```python
from build123d import *

# Parameters (mm, degrees)
SKETCH1_R           = 2.6375
BOSS_EXTRUDE1_DEPTH = 4


with BuildPart() as part:
    # Sketch1 → Boss-Extrude1 (new body)
    with BuildSketch(Plane.XY.offset(4)):
        with BuildLine():
            Line((17.952113198, 57.448352953), (10.955070442, 79.331722279))
            ThreePointArc((10.955070442, 79.331722279), (10.929647665, 81.056262686), (11.867204342, 82.503906776))
            ThreePointArc((11.867204342, 82.503906776), (9.81999759, 91.182758949), (4.022786968, 84.407371171))
            Line((4.022786968, 84.407371171), (3.500292698, 83.52050233))
            Line((3.500292698, 83.52050233), (14.672653681, 49.728262883))
            Line((14.672653681, 49.728262883), (15.200071751, 48.596801815))
            ThreePointArc((15.200071751, 48.596801815), (23.810416572, 47.35893823), (20.452073098, 55.383392934))
            ThreePointArc((20.452073098, 55.383392934), (18.899078146, 56.049025475), (17.952113198, 57.448352953))
        make_face()
        with Locations((19.856196321, 50.419026825)):
            Circle(SKETCH1_R, mode=Mode.SUBTRACT)
        with Locations((8.640951758, 86.323762043)):
            Circle(SKETCH1_R, mode=Mode.SUBTRACT)
    extrude(amount=-BOSS_EXTRUDE1_DEPTH)


solid = part.part
```
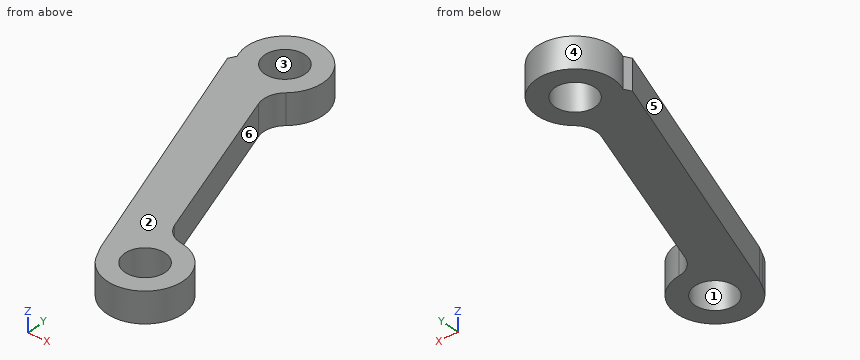
Verification items for the finished model (mm, model axes). Face numbers are marked on the shaded views. A direction names the side the tool comes from. Give positions to 0.01 mm unless a question says otherwise; leave off trailing zeros. Order: outer loops, then holes, each group sorted by start corner. A loop starts at its lowest first (then second) coordinate and runs counter-clockwise, first axis right, second up. Notation, with made-up numbers: M 14,17.5 L 35,17.5 A8 cw 35,26.5 Z; hole C -32.5,4.25 d4. An arc over 180 degrees is marked long. Return JSON: item names as keys, results as strings. Group by question number.
1) Section check C-C on z = 3. Record the cut outline in (x, y) (1 decimal).
2) Go/stop test with flat-tipped pins: pin 1 Ø1.5 at (y, z) = (55.5, 3) entering from -X; pin 2 Ø1.5 at (y, z) = (70.5, 2) entering from -X; pin 3 Ø1.5 at (y, z) = (64, 2) entering from +X. Record where each tip stops, or that it passes through.
3) Mould release check, pull along X, two halves, no side actions. Record for the marked faces 1, 2, 3 and 4: pulls with the +X half, pulls with the -X half, needs draft (parallel to the pull), parting line crosses it, or undercut.
4) Section check D-D on y = 58.5. Record the cut outline in (x, z).
5) Section check A-A on x = 13. Record the cut outline in (y, z), and give its area (3 significant figures).
6) Section check B-B on y = 85.5. Record the cut outline in (x, z).
7) Access from +Z, -Z, +X, -X, +Y, -Y to the whole of each face (thin tool, end or side, straight path). Record for the marked faces 5 and 6.
8) Scan lines: line 1 (X direction, y = 86.5, z = 2.4); line 2 (X direction, y = 85, z = 2); line 3 (Y direction, x = 18.75, z = 3.7). Record each from-to range of solid material in increasing order.
Answer block:
{
 "1": {"outline": "M 3.5,83.5 L 14.7,49.7 L 15.2,48.6 A5 ccw long 20.5,55.4 A3 cw 18,57.4 L 11,79.3 A3 cw 11.9,82.5 A5 ccw long 4,84.4 Z; hole C 8.6,86.3 d5.3; hole C 19.9,50.4 d5.3"},
 "2": {"pin 1": "stops at x = 12.52", "pin 2": "stops at x = 7.56", "pin 3": "stops at x = 16.1"},
 "3": {"face 1": "undercut", "face 2": "needs draft", "face 3": "undercut", "face 4": "parting line crosses it"},
 "4": {"outline": "M 11.77,0 L 17.62,0 L 17.62,4 L 11.77,4 Z"},
 "5": {"outline": "M 54.79,0 L 72.94,0 L 72.94,4 L 54.79,4 Z; M 83.87,0 L 88.77,0 L 88.77,4 L 83.87,4 Z", "area": "92.2 mm^2"},
 "6": {"outline": "M 3.71,0 L 6.14,0 L 6.14,4 L 3.71,4 Z; M 11.15,0 L 13.57,0 L 13.57,4 L 11.15,4 Z"},
 "7": {"face 5": "+Z, -Z, -X, -Y", "face 6": "+Z, -Z, +X"},
 "8": {"line 1": "x = 3.64 to 6.01, 11.27 to 13.64", "line 2": "x = 3.82 to 6.36, 10.92 to 13.46", "line 3": "y = 45.54 to 48.02, 52.81 to 56.18"}
}
